Verification items for the finished model (mm, model axes). Face numbers are marked on the shaded views. Round coordinates to 2 decimals unless told otherwise and drop trailing zeros. Order: outer loops, then holes, each group sorted by start corner. A loop starts at its lowest first (then second) coordinate and runs counter-clockwise, first axis right, second up. Notation, with made-up numbers: (14, 71.25) -> (62, 71.25) arc R15 ccw to (62, 89.25) -> close; hole circle Ø10 at (64, 57.25). An arc over 180 degrees is marked (long way). Answer in a Markdown table with one row per item. Add a question column.
```python
from build123d import *

# Parameters (mm, degrees)
SKETCH112_R     = 4
SKETCH112_R_2   = 1.6
PAD058_DEPTH    = 8
CHAMFER039_SIZE = 1.8
CHAMFER040_SIZE = 0.4


with BuildPart() as part:
    # Sketch112 → Pad058 (new body)
    with BuildSketch(Plane.YZ):
        Circle(SKETCH112_R)
        Circle(SKETCH112_R_2, mode=Mode.SUBTRACT)
    extrude(amount=PAD058_DEPTH)

    # Chamfer039
    chamfer039_edges = [part.edges().sort_by_distance(p)[0] for p in [
        (0, -1.6, 0),
    ]]
    chamfer(chamfer039_edges, length=CHAMFER039_SIZE)

    # Chamfer040
    chamfer040_edges = [part.edges().sort_by_distance(p)[0] for p in [
        (0, -4, 0),
        (8, -4, 0),
        (8, -1.6, 0),
    ]]
    chamfer(chamfer040_edges, length=CHAMFER040_SIZE)


with BuildPart() as part_1:
    # Body045 placement: moved
    add(part.part.moved(Location((-38, -48, 34.5))))


solid = part_1.part
```
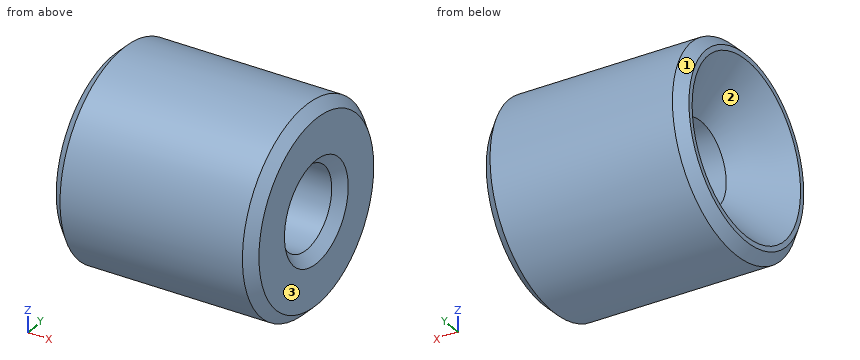
1) Cross-section at C-C, the plane x = -32.5. Record the boundary of the cut face in (y, z), and give its area (3 significant figures).
2) Thickness scan on L1, parallel to Z at x = -34.5, y = -48; L2, parallel to Y at x = -36.5, z = 33.5; L3, parallel to Y at x = -31.5, z = 34.75. Record the ranges inside material, lowest first. Write a range as [from, to].
3) Cross-section at A-A, the plane z = 34.5. Record the boundary of the cut face in (x, y).
4) Depth check by flat-ended pin: P1, Ø2, axis at y = -47, z = 34.5, coming from the -X side; P2, Ø1.5, axis at x = -37, y = -46.5, coming from the -Z side. Enter the tip coordinate at first touch or a pass-through.
5) Cross-section at B-B, the plane y = -48. Record the boundary of the cut face in (x, z).
6) Draft check along Y on the marked faces 1, 2 and 3. Enter one of: +Y half, -Y half, draft (parallel to the pull), parting line (faces both ways), or undercut.
Results below:
| question | item | result |
|---|---|---|
| 1 | outline | circle Ø8 at (-48, 34.5); hole circle Ø3.2 at (-48, 34.5) |
| 1 | area | 42.2 mm² |
| 2 | L1 | [30.5, 32.9], [36.1, 38.5] |
| 2 | L2 | [-51.87, -49.62], [-46.38, -44.13] |
| 2 | L3 | [-51.99, -49.58], [-46.42, -44.01] |
| 3 | outline | (-38, -51.6) -> (-37.6, -52) -> (-30.4, -52) -> (-30, -51.6) -> (-30, -50) -> (-30.4, -49.6) -> (-36.2, -49.6) -> (-38, -51.4) -> close; (-38, -44.6) -> (-36.2, -46.4) -> (-30.4, -46.4) -> (-30, -46) -> (-30, -44.4) -> (-30.4, -44) -> (-37.6, -44) -> (-38, -44.4) -> close |
| 4 | P1 | x = -36.6 |
| 4 | P2 | z = 30.57 |
| 5 | outline | (-38, 30.9) -> (-37.6, 30.5) -> (-30.4, 30.5) -> (-30, 30.9) -> (-30, 32.5) -> (-30.4, 32.9) -> (-36.2, 32.9) -> (-38, 31.1) -> close; (-38, 37.9) -> (-36.2, 36.1) -> (-30.4, 36.1) -> (-30, 36.5) -> (-30, 38.1) -> (-30.4, 38.5) -> (-37.6, 38.5) -> (-38, 38.1) -> close |
| 6 | face 1 | parting line |
| 6 | face 2 | undercut |
| 6 | face 3 | draft |
